Input: part model. Units: mm. Frame: model coordinates. A direction names the side the tool comes from. Give positions to 0.01 mm unless a question says otherwise; leave off trailing zeros. Loops run counter-clockwise (first coordinate to the right, second up) from the corner with the lowest first, then second, coordinate; pieces in that order, holes last. Notation, with made-up numbers: (53, 78) -> (96, 78) arc R27 cw to (96, 105) -> close; hole circle Ø6 at (13, 42). An arc over 180 degrees is marked (long way). Answer as a JSON object with one key per item and string values.
```python
from build123d import *

# Parameters (mm, degrees)
CROQUIS1_W                   = 19
CROQUIS1_H                   = 25.75
CROQUIS1_R                   = 1.000000029
CROQUIS1_R_2                 = 0.999999792
CROQUIS1_R_3                 = 1.000000052
CROQUIS1_R_4                 = 1.000000059
SALIENTE_EXTRUIR1_DEPTH      = 3
SALIENTE_EXTRUIR2_DEPTH      = 8
SALIENTE_EXTRUIR2_DEPTH_BACK = 8


with BuildPart() as part:
    # Croquis1 → Saliente-Extruir1 (new body)
    with BuildSketch(Plane(origin=(0, 0, 0), x_dir=(1, 0, 0), z_dir=(0, 1, 0))):
        with Locations((-0.226911439, -0.113455719)):
            Rectangle(CROQUIS1_W, CROQUIS1_H)
        with Locations((-6.226911361, 9.506544208)):
            Circle(CROQUIS1_R, mode=Mode.SUBTRACT)
        with Locations((5.773088267, 9.506544313)):
            Circle(CROQUIS1_R_2, mode=Mode.SUBTRACT)
        with Locations((5.773088494, -9.733455829)):
            Circle(CROQUIS1_R_3, mode=Mode.SUBTRACT)
        with Locations((-6.226911268, -9.733455698)):
            Circle(CROQUIS1_R_4, mode=Mode.SUBTRACT)
    extrude(amount=SALIENTE_EXTRUIR1_DEPTH)

    # Croquis2 → Saliente-Extruir2 (add, two sides)
    with BuildSketch(Plane.XY) as saliente_extruir2_sk:
        with BuildLine():
            Line((-3.708099244, 3), (3.708099244, 3))
            ThreePointArc((3.708099244, 3), (0, 5.5), (-3.708099244, 3))
        make_face()
    extrude(amount=SALIENTE_EXTRUIR2_DEPTH)
    extrude(saliente_extruir2_sk.sketch, amount=-SALIENTE_EXTRUIR2_DEPTH_BACK)


solid = part.part
```
Q1. Section B-B, the plane z = -0.75. Return the cut outline in (x, y).
Evaluation:
{"outline": "(-9.73, 0) -> (9.27, 0) -> (9.27, 3) -> (3.71, 3) arc R4 ccw to (-3.71, 3) -> (-9.73, 3) -> close"}
Q2. Ray query, line 1 along X through (y, z) = (2.6, 9.5); line 2 along Y through (x, z) = (2.5, 10.5); line 3 along Z through (x, y) = (-6.5, 2). Return the intervals inside material, ascending.
Evaluation:
{"line 1": "x = -9.73 to -7.2, -5.25 to 4.8, 6.75 to 9.27", "line 2": "y = 0 to 3", "line 3": "z = -12.76 to -10.47, -8.54 to 8.77, 10.7 to 12.99"}
Q3. Section A-A, the plane x = -6. Return the cut outline in (y, z), then the cut area to 3 significant figures.
Evaluation:
{"outline": "(0, -12.76) -> (3, -12.76) -> (3, -10.48) -> (0, -10.48) -> close; (0, -8.53) -> (3, -8.53) -> (3, 8.76) -> (0, 8.76) -> close; (0, 10.71) -> (3, 10.71) -> (3, 12.99) -> (0, 12.99) -> close", "area": "65.6 mm2"}
Q4. Pin query (flat end, axial travel): pin 1 (1.6 mm diameter, centred on x = 5.77, z = 9.73, fed in from +Y); pin 2 (2.5 mm diameter, centred on x = -6.23, z = 9.73, fed in from +Y); pin 3 (0.8 mm diameter, centred on x = -0.5, y = 4.5, fed in from +Z); pin 4 (1.2 mm diameter, centred on x = -1, y = 4.5, fed in from -Z). Return the tip coordinate at first contact, or that it passes through.
Evaluation:
{"pin 1": "passes through", "pin 2": "stops at y = 3", "pin 3": "stops at z = 8", "pin 4": "stops at z = -8"}
Q5. Draft query along Z for faces 3 (the flat face through (0, 4, -8)), 4 (the cylindrical face through (-6.44, 1.48, -8.53)), 5 (the flat face through (0, 1, 12.988)), 6 (the flat face through (-9.727, 1, 0)). Return one class per face: +Z half, -Z half, draft (parallel to the pull), parting line (faces both ways), or undercut.
Evaluation:
{"face 3": "-Z half", "face 4": "undercut", "face 5": "+Z half", "face 6": "draft"}
Q6. Access query for faces 1 (the flat face through (0, 4, 8)), 2 (the flat face through (0, 1, -12.762)). Directions: +Z, -Z, +X, -X, +Y, -Y. A direction counts if a zero-diameter tool reaches every point of the face in a straight line with its end or side. Return the directions, or none.
Evaluation:
{"face 1": "+Z, +X, -X, +Y", "face 2": "-Z, +X, -X, +Y, -Y"}
Q7. Section C-C, the plane x = -2.25. Return the cut outline in (y, z), then the cut area to 3 significant figures.
Evaluation:
{"outline": "(0, -12.76) -> (3, -12.76) -> (3, -8) -> (4.81, -8) -> (4.81, 8) -> (3, 8) -> (3, 12.99) -> (0, 12.99) -> close", "area": "106 mm2"}
Q8. Section D-D, the plane y = 2.2. Return the cut outline in (x, z), then the cut area to 3 significant figures.
Evaluation:
{"outline": "(-9.73, -12.76) -> (9.27, -12.76) -> (9.27, 12.99) -> (-9.73, 12.99) -> close; hole circle Ø2 at (-6.23, -9.51); hole circle Ø2 at (-6.23, 9.73); hole circle Ø2 at (5.77, -9.51); hole circle Ø2 at (5.77, 9.73)", "area": "477 mm2"}
